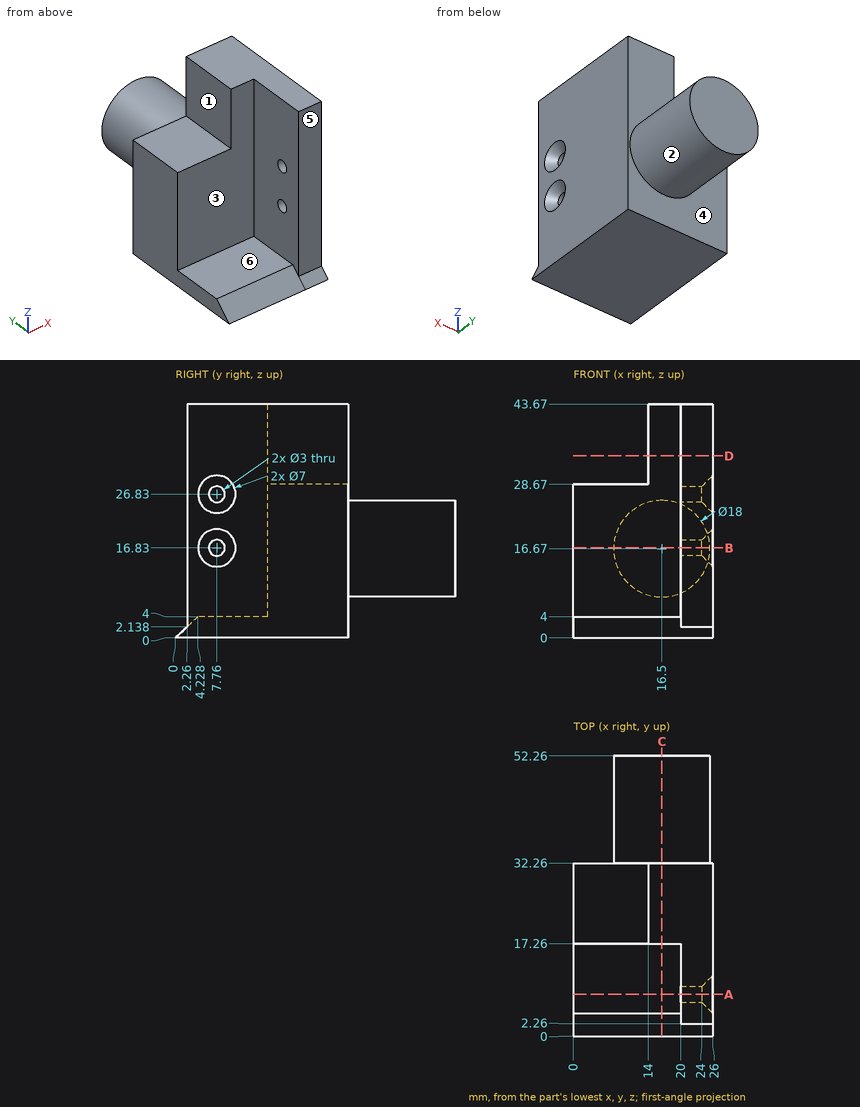
Here's the drawing with two shaded views (mm, measured from the low corner). I have some questions. A direction names the side the tool comes from. Give positions to 0.01 mm unless a question says otherwise; leave off trailing zeros. Order: outer loops, then holes, each group sorted by start corner. A loop starts at its lowest first (then second) coordinate and runs counter-clockwise, first axis right, second up. Notation, with made-up numbers: (-28, 21) -> (-23, 21) arc R25 cw to (-23, 58) -> close; hole circle Ø8 at (-15.75, 75.25). An arc over 180 degrees is marked (long way). One line per item, written item: value. Start each with the question number.
1. We'd pull the mould along Y, two halves only. Please class the marked faces 4, 5 and 6: released by +Y, released by -Y, zero draft, split by the parting line, or undercut.
2. Imagine slicing it at D-D, the plane z = 34. List the corners of the cut face in (x, y) for me.
3. I need wall thicknesses on probe 1 along Y at (x, z) = (21, 26.83); probe 2 along Y at (x, z) = (22.6, 16.83); probe 3 along Z at (x, y) = (9, 18.5). Which ranges of each line are inside material? Lowest first, please. Write a range as from..to.
4. Imagine slicing it at B-B, the plane z = 16.83. List the corners of the cut face in (x, y) for me.
5. Imagine slicing it at A-A, the plane y = 7.76. List the corners of the cut face in (x, z) for me.
6. Imagine slicing it at C-C, the plane x = 16.5. List the corners of the cut face in (y, z) for me, plus the area to 3 significant figures.
7. Will these pins go through, and if not, where does the flat tip stop? pin 1 Ø4 at (x, y) = (20.5, 5.5) entering from -Z; pin 2 Ø1.5 at (x, z) = (19.5, 8.5) entering from -Y; pin 3 Ø7.5 at (y, z) = (11, 12.5) entering from -X; pin 4 Ø11 at (x, y) = (6.5, 27) entering from +Z.
8. For the marked faces 1, 2 and 3, which set-ups out of +Z, -Z, +X, -X, +Y, -Y let a thin tool reach every point of the face, with its end or its side?
Values follow:
1. face 4: released by +Y
1. face 5: released by -Y
1. face 6: zero draft
2. outline: (14, 17.26) -> (20, 17.26) -> (20, 2.26) -> (26, 2.26) -> (26, 32.26) -> (14, 32.26) -> close
3. probe 1: y = 2.26..6.26, 9.26..32.26
3. probe 2: y = 2.26..6.26, 9.26..52.26
3. probe 3: z = 0..28.67
4. outline: (0, 17.26) -> (20, 17.26) -> (20, 9.26) -> (24, 9.26) -> (26, 11.26) -> (26, 32.26) -> (25.5, 32.26) -> (25.5, 52.26) -> (7.5, 52.26) -> (7.5, 32.26) -> (0, 32.26) -> close; (20, 2.26) -> (26, 2.26) -> (26, 4.26) -> (24, 6.26) -> (20, 6.26) -> close
5. outline: (0, 0) -> (26, 0) -> (26, 13.33) -> (24, 15.33) -> (20, 15.33) -> (20, 4) -> (0, 4) -> close; (20, 18.33) -> (24, 18.33) -> (26, 20.33) -> (26, 23.33) -> (24, 25.33) -> (20, 25.33) -> close; (20, 28.33) -> (24, 28.33) -> (26, 30.33) -> (26, 43.67) -> (20, 43.67) -> close
6. outline: (0, 0) -> (32.26, 0) -> (32.26, 7.67) -> (52.26, 7.67) -> (52.26, 25.67) -> (32.26, 25.67) -> (32.26, 43.67) -> (17.26, 43.67) -> (17.26, 4) -> (4.23, 4) -> close
6. area: 1,080 mm2
7. pin 1: stops at z = 0
7. pin 2: stops at y = 2.26
7. pin 3: stops at x = 20
7. pin 4: stops at z = 28.67
8. face 1: +Z, -X, +Y, -Y
8. face 2: +Y
8. face 3: +Z, -X, -Y
